from build123d import *

# Parameters (mm, degrees)
F0_W     = 127
F0_H     = 44.45
F1_DEPTH = 6.35
F2_R     = 5.08
F3_R     = 6.35
F4_DEPTH = 6.35


with BuildPart() as f1:
    # F0 (on Top) → F1 (new body)
    with BuildSketch(Plane.XY):
        Rectangle(F0_W, F0_H)
    extrude(amount=F1_DEPTH)

    # F2
    f2_edges = [f1.edges().sort_by_distance(p)[0] for p in [
        (63.5, -22.225, 3.175),
        (63.5, 22.225, 3.175),
        (-63.5, -22.225, 3.175),
        (-63.5, 22.225, 3.175),
    ]]
    fillet(f2_edges, radius=F2_R)

    # F3 (on face) → F4 (cut, through all)
    with BuildSketch(Plane.XY.offset(6.35)):
        with Locations((-44.45, 0)):
            Circle(F3_R)
        with Locations((44.45, 0)):
            Circle(F3_R)
    extrude(amount=-F4_DEPTH, mode=Mode.SUBTRACT)


solid = f1.part
Part model, mm, in its own coordinate system. Round coordinates to 2 decimals unless told otherwise and drop trailing zeros. Loops run counter-clockwise (first coordinate to the right, second up) from the corner with the lowest first, then second, coordinate; pieces in that order, holes last. Notation, with made-up numbers: (-31, 9) - (27, 9) arc R10 cw to (27, 17) - close; hole circle Ø2 at (57.25, 15.25). An arc over 180 degrees is marked (long way). Answer as a JSON object with one key per item and string values.
Item 1: Band-saw the part on D-D on x = -43.5. List the corners of the cut face in (y, z) (3 decimals).
Output:
{"outline": "(-22.225, 0) - (-6.279, 0) - (-6.279, 6.35) - (-22.225, 6.35) - close; (6.279, 0) - (22.225, 0) - (22.225, 6.35) - (6.279, 6.35) - close"}
Item 2: Band-saw the part on C-C on z = 1.75. List the corners of the cut face in (x, y) (3 decimals).
Output:
{"outline": "(-63.5, -17.145) arc R5.08 ccw to (-58.42, -22.225) - (58.42, -22.225) arc R5.08 ccw to (63.5, -17.145) - (63.5, 17.145) arc R5.08 ccw to (58.42, 22.225) - (-58.42, 22.225) arc R5.08 ccw to (-63.5, 17.145) - close; hole circle Ø12.7 at (-44.45, 0); hole circle Ø12.7 at (44.45, 0)"}
Item 3: Band-saw the part on B-B on x = 44.45. List the corners of the cut face in (y, z) (3 decimals), plus the area to 3 significant figures.
Output:
{"outline": "(-22.225, 0) - (-6.35, 0) - (-6.35, 6.35) - (-22.225, 6.35) - close; (6.35, 0) - (22.225, 0) - (22.225, 6.35) - (6.35, 6.35) - close", "area": "202 mm2"}
Item 4: Pull direction Y, two halves, no side cores. Call faces 1 (the face through (-1, 0, 0)), 2 (the face through (-38.393, 1.907, 3.219)), 3 (the face through (-1, -22.225, 3)): pulls with the +Y half, pulls with the -Y half, needs draft (parallel to the pull), parting line crosses it, or undercut.
Output:
{"face 1": "needs draft", "face 2": "undercut", "face 3": "pulls with the -Y half"}
Item 5: Band-saw the part on A-A on y = 0. List the corners of the cut face in (x, z), plus the area to 3 significant figures.
Output:
{"outline": "(-63.5, 0) - (-50.8, 0) - (-50.8, 6.35) - (-63.5, 6.35) - close; (-38.1, 0) - (38.1, 0) - (38.1, 6.35) - (-38.1, 6.35) - close; (50.8, 0) - (63.5, 0) - (63.5, 6.35) - (50.8, 6.35) - close", "area": "645 mm2"}
Item 6: Wall check: L1, parallel to X at y = -0.5, z = 3.75; L2, parallel to Y at x = 44.45, z = 4.5 (3 decimals); L3, parallel to X at y = 1, z = 1. Give the ranges that are in metal, low to high.
Output:
{"L1": "-63.5 to -50.78, -38.12 to 38.12, 50.78 to 63.5", "L2": "-22.225 to -6.35, 6.35 to 22.225", "L3": "-63.5 to -50.72, -38.18 to 38.18, 50.72 to 63.5"}
